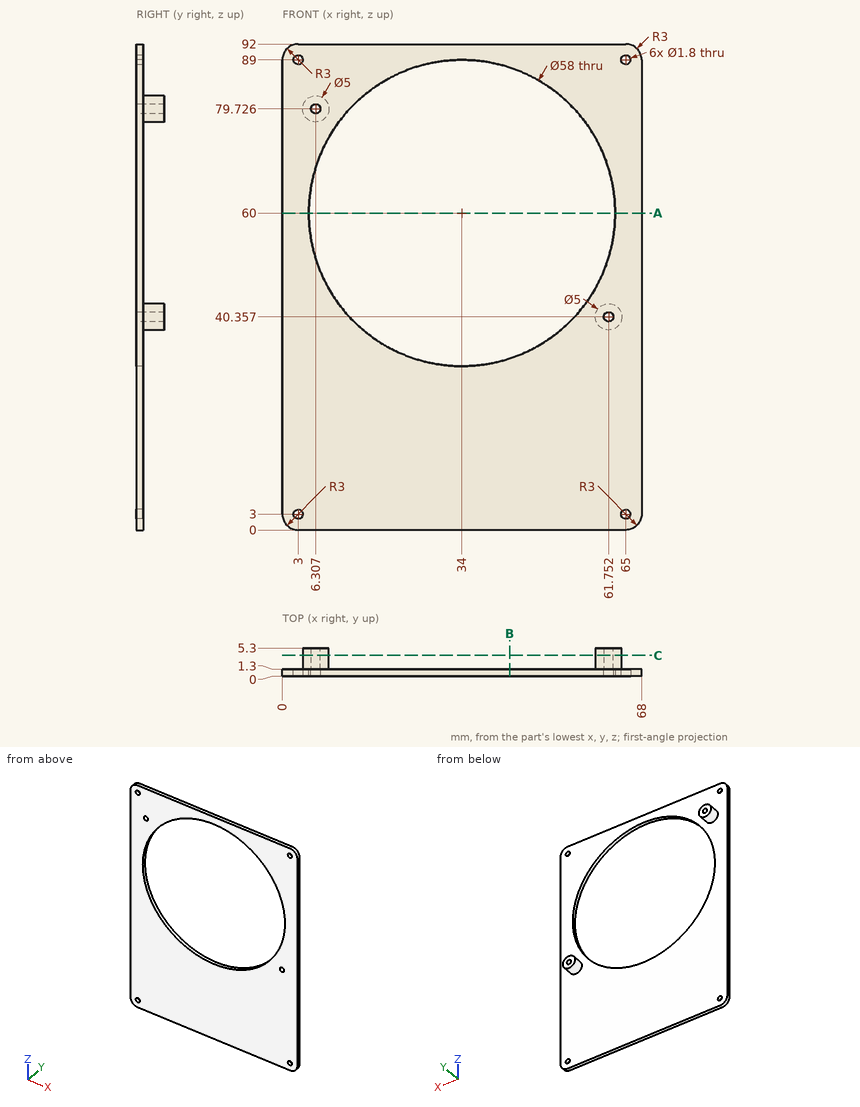
Print and shaded views of the part. All mm, measured from the part's lowest x, y and z. Give positions to 0.01 mm unless a question says otherwise; leave off trailing zeros. Order: outer loops, then holes, each group sorted by start corner. A loop starts at its lowest first (then second) coordinate and runs counter-clockwise, first axis right, second up. Notation, with made-up numbers: (38, 38.25) - (58, 38.25) arc R21 cw to (58, 50.25) - close; hole circle Ø4 at (-33.75, -1.75). An arc over 180 degrees is marked (long way). One line per item, written item: value.
Item 1: Pin check, flat tip, straight feed: pin 1 Ø1 at (x, z) = (21.5, 9) entering from +Y. Stop position of the tip, or through.
Response values:
pin 1: y = 1.3
Item 2: Slice it at B-B (x = 43). List the corners of the cut face in (y, z).
Response values:
outline: (0, 0) - (1.3, 0) - (1.3, 32.43) - (0, 32.43) - close; (0, 87.57) - (1.3, 87.57) - (1.3, 92) - (0, 92) - close
Item 3: Slice it at A-A (z = 60). List the corners of the cut face in (x, y), then the cut area to 3 significant figures.
Response values:
outline: (0, 0) - (5, 0) - (5, 1.3) - (0, 1.3) - close; (63, 0) - (68, 0) - (68, 1.3) - (63, 1.3) - close
area: 13.0 mm2
Item 4: Slice it at C-C (y = 3.9). List the corners of the cut face in (x, z).
Response values:
outline: circle Ø5 at (6.31, 79.73); circle Ø5 at (61.75, 40.36); hole circle Ø1.8 at (6.31, 79.73); hole circle Ø1.8 at (61.75, 40.36)
Item 5: Wall check: line 1 (Z direction, x = 65, y = 0.95); line 2 (Y direction, x = 60, z = 34.5); line 3 (Z direction, x = 22.5, y = 1). Give the ranges that are in metal, low to high.
Response values:
line 1: 0 to 2.1, 3.9 to 88.1, 89.9 to 92
line 2: 0 to 1.3
line 3: 0 to 33.38, 86.62 to 92
